```python
from build123d import *

# Parameters (mm, degrees)
SKETCH1_W               = 17
SKETCH1_H               = 20
BOSS_EXTRUDE1_DEPTH     = 20
SKETCH2_W               = 13
SKETCH2_H               = 18
CUT_EXTRUDE1_DEPTH      = 18
CUT_EXTRUDE2_DEPTH      = 1
CUT_EXTRUDE2_DEPTH_BACK = 18
CUT_EXTRUDE3_REACH      = 4
CUT_EXTRUDE4_REACH      = 4
BOSS_EXTRUDE2_DEPTH     = 1
BOSS_EXTRUDE3_DEPTH     = 1


with BuildPart() as part:
    # Sketch1 → Boss-Extrude1 (new body)
    with BuildSketch(Plane.XY):
        Rectangle(SKETCH1_W, SKETCH1_H)
    extrude(amount=BOSS_EXTRUDE1_DEPTH)

    # Sketch2 → Cut-Extrude1 (cut)
    with BuildSketch(Plane(origin=(0, 10, 0), x_dir=(1, 0, 0), z_dir=(0, 1, 0))):
        with Locations((0, -11)):
            Rectangle(SKETCH2_W, SKETCH2_H)
    extrude(amount=-CUT_EXTRUDE1_DEPTH, mode=Mode.SUBTRACT)

    # Sketch3 → Cut-Extrude2 (cut, two sides)
    with BuildSketch(Plane(origin=(8.5, 0, 0), x_dir=(0, 0, -1), z_dir=(1, 0, 0))) as cut_extrude2_sk:
        Polygon((-2, 10), (-20, -8), (-20, 10), align=None)
    extrude(amount=CUT_EXTRUDE2_DEPTH, mode=Mode.SUBTRACT)
    extrude(cut_extrude2_sk.sketch, amount=-CUT_EXTRUDE2_DEPTH_BACK, mode=Mode.SUBTRACT)

    # Sketch4 → Cut-Extrude3 (cut, up to next)
    with BuildSketch(Plane(origin=(0, -8, 0), x_dir=(1, 0, 0), z_dir=(0, 1, 0)), mode=Mode.PRIVATE) as cut_extrude3_sk1:
        with BuildLine():
            Line((-3, -12), (-3, -7))
            ThreePointArc((-3, -7), (0, -4), (3, -7))
            Line((3, -7), (3, -12))
            ThreePointArc((3, -12), (0, -15), (-3, -12))
        make_face()
    cut_extrude3_tool1 = extrude(cut_extrude3_sk1.sketch, amount=-CUT_EXTRUDE3_REACH, mode=Mode.PRIVATE) & part.part
    add(cut_extrude3_tool1.solids().sort_by_distance((0, -8, 9.5))[0], mode=Mode.SUBTRACT)

    # Sketch5 → Cut-Extrude4 (cut, up to next)
    with BuildSketch(Plane.XY.offset(2), mode=Mode.PRIVATE) as cut_extrude4_sk1:
        with BuildLine():
            Line((-3, -3), (-3, 2))
            ThreePointArc((-3, 2), (0, 5), (3, 2))
            Line((3, 2), (3, -3))
            ThreePointArc((3, -3), (0, -6), (-3, -3))
        make_face()
    cut_extrude4_tool1 = extrude(cut_extrude4_sk1.sketch, amount=-CUT_EXTRUDE4_REACH, mode=Mode.PRIVATE) & part.part
    add(cut_extrude4_tool1.solids().sort_by_distance((0, -0.5, 2))[0], mode=Mode.SUBTRACT)

    # Sketch6 → Boss-Extrude2 (add)
    with BuildSketch(Plane.XZ.offset(10)):
        with BuildLine():
            Line((-1, 19), (1, 19))
            ThreePointArc((1, 19), (2, 18), (1, 17))
            Line((1, 17), (-1, 17))
            ThreePointArc((-1, 17), (-2, 18), (-1, 19))
        make_face()
        with BuildLine():
            Line((-1, 3), (1, 3))
            ThreePointArc((1, 3), (2, 2), (1, 1))
            Line((1, 1), (-1, 1))
            ThreePointArc((-1, 1), (-2, 2), (-1, 3))
        make_face()
    extrude(amount=BOSS_EXTRUDE2_DEPTH)

    # Sketch7 → Boss-Extrude3 (add)
    with BuildSketch(Plane(origin=(0, 0, 0), x_dir=(-1, 0, 0), z_dir=(0, 0, -1))):
        with BuildLine():
            Line((1, -9), (-1, -9))
            ThreePointArc((-1, -9), (-2, -8), (-1, -7))
            Line((-1, -7), (1, -7))
            ThreePointArc((1, -7), (2, -8), (1, -9))
        make_face()
        with BuildLine():
            Line((1, 7), (-1, 7))
            ThreePointArc((-1, 7), (-2, 8), (-1, 9))
            Line((-1, 9), (1, 9))
            ThreePointArc((1, 9), (2, 8), (1, 7))
        make_face()
    extrude(amount=BOSS_EXTRUDE3_DEPTH)


solid = part.part
```
Verification items for the finished model (mm, model axes). A direction names the side the tool comes from. Round coordinates to 2 decimals unless told otherwise and drop trailing zeros. Write each loop counter-clockwise with the first axis right and the second up, starting at its lowest first coordinate (ties: lowest second). Pieces come first, ordered by that corner, then holes.
1. Section check B-B on z = 7.75. Enter the section's corners in (x, y).
2. Section check A-A on y = -1. Enter the section's corners in (x, z).
3. Access from +Z, -Z, +X, -X, +Y, -Y to the whole of each face (thin tool, end or side, straight path). Record for faces 1 (the cylindrical face through (0, -9, 4)), 2 (the flat face through (3, 0, 1)), 3 (the cylindrical face through (2, -10.5, 2)), 4 (the flat face through (-3, 3, 2)).
4. Draft check along Z on faces 5 (the cylindrical face through (-2, 8, -0.5)), 6 (the flat face through (0, -9, 20)), 7 (the flat face through (-3, -9, 10)), 8 (the flat face through (0, -10.5, 3)). Enter one of: +Z half, -Z half, draft (parallel to the pull), parting line (faces both ways), or undercut.
5. Section check C-C on x = 7.5. Enter the section's corners in (y, z), plus the area to 3 significant figures.
6. Scan lines: L1, parallel to X at y = -9, z = 7; L2, parallel to X at y = 1.25, z = 6; L3, parallel to Z at x = 6, y = -4. Record each from-to range of solid material in increasing order.
7. Section check D-D on y = 8. Enter the section's corners in (x, z), plus the area to 3 significant figures.
8. Gauge pin test, flat ends, axial feed: P1, Ø4, axis at x = 5.5, y = 4, coming from the -Z side; P2, Ø1.1, axis at x = 0, z = -0.5, coming from the +Y side; P3, Ø1, axis at x = -5.5, z = 13.5, coming from the -Y side; P4, Ø2, axis at x = 6, y = -1, coming from the +Z side. Record the tip position at first contact, or that the pin passes through.
Answer:
1. outline: (-8.5, -10) - (-3, -10) - (-3, -8) - (-6.5, -8) - (-6.5, 4.25) - (-8.5, 4.25) - close; (3, -10) - (8.5, -10) - (8.5, 4.25) - (6.5, 4.25) - (6.5, -8) - (3, -8) - close
2. outline: (-8.5, 0) - (-3, 0) - (-3, 2) - (-6.5, 2) - (-6.5, 13) - (-8.5, 13) - close; (3, 0) - (8.5, 0) - (8.5, 13) - (6.5, 13) - (6.5, 2) - (3, 2) - close
3. face 1: +Y, -Y
3. face 2: +Z, -Z
3. face 3: +X, -Y
3. face 4: +Z, +Y
4. face 5: draft
4. face 6: +Z half
4. face 7: undercut
4. face 8: undercut
5. outline: (-10, 0) - (10, 0) - (10, 2) - (-8, 20) - (-10, 20) - close
5. area: 238 mm2
6. L1: x = -8.5 to -3, 3 to 8.5
6. L2: x = -8.5 to -6.5, 6.5 to 8.5
6. L3: z = 0 to 2
7. outline: (-8.5, 0) - (-2, 0) - (-2, -1) - (2, -1) - (2, 0) - (8.5, 0) - (8.5, 4) - (6.5, 4) - (6.5, 2) - (-6.5, 2) - (-6.5, 4) - (-8.5, 4) - close
7. area: 46.0 mm2
8. P1: stops at z = 0
8. P2: stops at y = 10
8. P3: stops at y = -10
8. P4: stops at z = 13.87
